```python
from build123d import *

# Parameters (mm, degrees)
SKETCH2_W                    = 64.5
SKETCH2_H                    = 64.5
BOSS_EXTRUDE1_DEPTH          = 2
SKETCH3_W                    = 7
SKETCH3_H                    = 7
BOSS_EXTRUDE2_DEPTH          = 10
SKETCH6_R                    = 1
CUT_EXTRUDE2_DEPTH           = 3
CHAMFER3_SIZE                = 3
CIRPATTERN1_COUNT            = 3
CIRPATTERN1_ANGLE            = 180
CHAMFER3_OF_CIRPATTERN1_SIZE = 3
CHAMFER8_SIZE                = 4
FILLET4_R                    = 0.5
SKETCH12_W                   = 15
SKETCH12_H                   = 3
CUT_EXTRUDE3_DEPTH           = 10
CHAMFER9_SIZE                = 1
SKETCH13_R                   = 3.75
CUT_EXTRUDE4_DEPTH           = 10
SKETCH16_R                   = 1.25
CUT_EXTRUDE6_DEPTH           = 10
CHAMFER10_SIZE               = 1
CHAMFER10_SIZE2              = 0.700207538


with BuildPart() as part:
    # Sketch2 → Boss-Extrude1 (new body)
    with BuildSketch(Plane(origin=(0, 0, 0), x_dir=(1, 0, 0), z_dir=(0, 1, 0))):
        Rectangle(SKETCH2_W, SKETCH2_H)
    extrude(amount=BOSS_EXTRUDE1_DEPTH)

    # Sketch3 → Boss-Extrude2 (add)
    with BuildSketch(Plane.XZ):
        with Locations((-28.75, 28.75)):
            Rectangle(SKETCH3_W, SKETCH3_H)
    boss_extrude2 = extrude(amount=BOSS_EXTRUDE2_DEPTH)

    # Sketch6 → Cut-Extrude2 (cut)
    with BuildSketch(Plane.XZ.offset(10)):
        with Locations((-28.75, 28.75)):
            Circle(SKETCH6_R)
    cut_extrude2 = extrude(amount=-CUT_EXTRUDE2_DEPTH, mode=Mode.SUBTRACT)

    # Chamfer3
    chamfer3_edges = [part.edges().sort_by_distance(p)[0] for p in [
        (-28.75, 0, 25.25),
        (-25.25, 0, 28.75),
    ]]
    chamfer(chamfer3_edges, length=CHAMFER3_SIZE)

    # CirPattern1: Boss-Extrude2, Cut-Extrude2 ×3 about axis
    cirpattern1_axis = Axis((0, 0, 0), (0, -1, 0))
    for i in range(1, CIRPATTERN1_COUNT):
        add(boss_extrude2.rotate(cirpattern1_axis, i * CIRPATTERN1_ANGLE / (CIRPATTERN1_COUNT - 1)))
        add(cut_extrude2.rotate(cirpattern1_axis, i * CIRPATTERN1_ANGLE / (CIRPATTERN1_COUNT - 1)), mode=Mode.SUBTRACT)

    # Chamfer3 of CirPattern1
    chamfer3_of_cirpattern1_edges = [part.edges().sort_by_distance(p)[0] for p in [
        (-25.25, 0, -28.75),
        (-28.75, 0, -25.25),
        (28.75, 0, -25.25),
        (25.25, 0, -28.75),
    ]]
    chamfer(chamfer3_of_cirpattern1_edges, length=CHAMFER3_OF_CIRPATTERN1_SIZE)

    # Chamfer8
    chamfer8_edges = [part.edges().sort_by_distance(p)[0] for p in [
        (32.25, 1, 32.25),
        (-32.25, -4, 32.25),
        (-32.25, -4, -32.25),
        (32.25, -4, -32.25),
    ]]
    chamfer(chamfer8_edges, length=CHAMFER8_SIZE)

    # Fillet4
    fillet4_edges = [part.edges().sort_by_distance(p)[0] for p in [
        (30.25, 0, 30.25),
        (0, 2, 32.25),
        (-28.25, -4, 32.25),
        (28.25, 1, 32.25),
        (0, 2, -32.25),
        (-32.25, 2, 0),
        (-30.25, 2, 30.25),
        (-30.25, 2, -30.25),
        (30.25, 2, -30.25),
        (30.25, 2, 30.25),
        (-28.25, -4, -32.25),
        (28.25, -4, -32.25),
        (-32.25, -4, 28.25),
        (-32.25, -4, -28.25),
        (-32.25, -6.5, 25.25),
        (-25.25, -6.5, 25.25),
        (-25.25, -6.5, 32.25),
        (3, 0, 32.25),
        (-23.75, -1.5, 32.25),
        (-32.25, -1.5, 23.75),
        (-25.25, -6.5, -32.25),
        (-25.25, -6.5, -25.25),
        (-32.25, -6.5, -25.25),
        (32.25, -6.5, -25.25),
        (25.25, -6.5, -25.25),
        (25.25, -6.5, -32.25),
        (-32.25, 0, 0),
        (-32.25, -1.5, -23.75),
        (-23.75, -1.5, -32.25),
        (0, 0, -32.25),
        (23.75, -1.5, -32.25),
        (32.25, -1.5, -23.75),
        (32.25, 0, 3),
        (32.25, 2, 0),
        (32.25, -4, -28.25),
        (32.25, 1, 28.25),
    ]]
    fillet(fillet4_edges, radius=FILLET4_R)

    # Sketch12 → Cut-Extrude3 (cut)
    with BuildSketch(Plane(origin=(0, 2, 0), x_dir=(1, 0, 0), z_dir=(0, 1, 0))):
        with Locations((0, -30.75)):
            Rectangle(SKETCH12_W, SKETCH12_H)
    extrude(amount=-CUT_EXTRUDE3_DEPTH, mode=Mode.SUBTRACT)

    # Chamfer9
    chamfer9_edges = [part.edges().sort_by_distance(p)[0] for p in [
        (-7.5, 1, 29.25),
        (7.5, 1, 29.25),
    ]]
    chamfer(chamfer9_edges, length=CHAMFER9_SIZE)

    # Sketch13 → Cut-Extrude4 (cut)
    with BuildSketch(Plane(origin=(0, 2, 0), x_dir=(1, 0, 0), z_dir=(0, 1, 0))):
        with Locations((8.75, -23.5)):
            Circle(SKETCH13_R)
        with Locations((-8.75, -23.5)):
            Circle(SKETCH13_R)
        with Locations((-8.75, 23.5)):
            Circle(SKETCH13_R)
        with Locations((8.75, 23.5)):
            Circle(SKETCH13_R)
    extrude(amount=-CUT_EXTRUDE4_DEPTH, mode=Mode.SUBTRACT)

    # Sketch16 → Cut-Extrude6 (cut)
    with BuildSketch(Plane.XZ):
        with Locations((-27.25, -17.25)):
            Circle(SKETCH16_R)
        with Locations((-27.25, 17.25)):
            Circle(SKETCH16_R)
        with Locations((27.25, -17.25)):
            Circle(SKETCH16_R)
        with Locations((27.25, 17.25)):
            Circle(SKETCH16_R)
    extrude(amount=-CUT_EXTRUDE6_DEPTH, mode=Mode.SUBTRACT)

    # Chamfer10
    chamfer10_edges = [part.edges().sort_by_distance(p)[0] for p in [
        (-28.5, 0, 17.25),
        (26, 0, -17.25),
        (26, 0, 17.25),
        (-28.5, 0, -17.25),
    ]]
    chamfer10_side = [part.faces().sort_by_distance(p)[0] for p in [
        (0.632372559, 0, 0.31600784),
    ]]
    chamfer(chamfer10_edges, length=CHAMFER10_SIZE, length2=CHAMFER10_SIZE2, reference=chamfer10_side[0])


solid = part.part
```
Geometry check sheet. Reference: the model listing, model coordinates, mm. A direction names the side the tool comes from. Round coordinates to 2 decimals unless told otherwise and drop trailing zeros. Order: outer loops, then holes, each group sorted by start corner. A loop starts at its lowest first (then second) coordinate and runs counter-clockwise, first axis right, second up. Notation, with made-up numbers: (-1.75, 6.25) -> (47.25, 6.25) arc R11 cw to (47.25, 25.25) -> close; hole circle Ø7 at (64, 28). An arc over 180 degrees is marked (long way). Return JSON: item names as keys, results as strings. Group by question number.
Q1. Tool access check on faces 4 (the flat face through (25.25, -6, -29)), 5 (the flat face through (-29, -7, 29)), 6 (the flat face through (-29, -6, -25.25)). Record the directions out of +Z, -Z, +X, -X, +Y, -Y that give a thin tool (end or side, any length) a straight path to the whole face; none if there is none.
Q2. Section check B-B, the plane x = -8.75. Record the boundary of the cut face in (y, z).
Q3. Section check C-C, the plane z = 12. Record the boundary of the cut face in (x, y).
Q4. Material ranges on probe 1 along Z at (x, y) = (-8.75, 0.95); probe 2 along X at (y, z) = (-8.4, -28.75); probe 3 along X at (y, z) = (0.45, 23.5), recorded low to high. Write a range as from..to.
Q5. Section check D-D, the plane x = 16. Record the boundary of the cut face in (y, z), plus the area to 3 significant figures.
Q6. Release check for a two-part mould opening along X. For faces 1 (the cylindrical face through (7.94, 1.01, -19.84)), 2 (the cylindrical face through (30.12, 0.15, 30.18)), 3 (the flat face through (28, -10, -27)) record: released by +X, released by -X, zero draft, split by the parting line, or undercut.
Q7. Section check A-A, the plane y = -8.5. Count the separate pieces of the cut face and the enclosed holes in it, plus the area to 3 significant figures.
Q8. Gauge pin test, flat ends, axial feed: pin 1 (1 mm diameter, centred on x = -29, z = 29, fed in from -Y); pin 2 (8 mm diameter, centred on x = 24, z = 23.5, fed in from -Y); pin 3 (4 mm diameter, centred on x = -27.25, z = -17.25, fed in from -Y). Record the tip position at first contact, or that the pin passes through.
Numbers:
{
 "1": {"face 4": "+Z, -Z, -Y", "face 5": "-Y", "face 6": "+X, -X, -Y"},
 "2": {"outline": "(0, -31.75) arc R0.5 ccw to (0.5, -32.25) -> (1.5, -32.25) arc R0.5 ccw to (2, -31.75) -> (2, -27.25) -> (0, -27.25) -> close; (0, -19.75) -> (2, -19.75) -> (2, 19.75) -> (0, 19.75) -> close; (0, 27.25) -> (2, 27.25) -> (2, 31.75) arc R0.5 ccw to (1.5, 32.25) -> (0.5, 32.25) arc R0.5 ccw to (0, 31.75) -> close"},
 "3": {"outline": "(-32.25, 0.5) arc R0.5 ccw to (-31.75, 0) -> (31.75, 0) arc R0.5 ccw to (32.25, 0.5) -> (32.25, 1.5) arc R0.5 ccw to (31.75, 2) -> (-31.75, 2) arc R0.5 ccw to (-32.25, 1.5) -> close"},
 "4": {"probe 1": "-32.25..-27.25, -19.75..19.75, 27.25..32.25", "probe 2": "-31.75..-29.75, -27.75..-25.25, 25.25..27.75, 29.75..31.75", "probe 3": "-32.25..-12.5, -5..5, 12.5..32.25"},
 "5": {"outline": "(0, -31.75) arc R0.5 ccw to (0.5, -32.25) -> (1.5, -32.25) arc R0.5 ccw to (2, -31.75) -> (2, 31.75) arc R0.5 ccw to (1.5, 32.25) -> (0.5, 32.25) arc R0.5 ccw to (0, 31.75) -> close", "area": "129 mm^2"},
 "6": {"face 1": "undercut", "face 2": "released by +X", "face 3": "zero draft"},
 "7": {"separate pieces": "3", "enclosed holes": "3", "area": "113 mm^2"},
 "8": {"pin 1": "y = -7", "pin 2": "y = 0", "pin 3": "y = 0.18"}
}
